Autodesk Inventor part; units mm, degrees
ref_plane "YZ Plane" through (0, 0, 0) normal (1, 0, 0) x (0, 1, 0)
ref_plane "XZ Plane" through (0, 0, 0) normal (0, 1, 0) x (-1, 0, 0)
ref_plane "XY Plane" through (0, 0, 0) normal (0, 0, 1) x (1, 0, 0)
sketch "2020_Base" plane through (0, 0, 0) normal (0, 1, 0) x (-1, 0, 0)
  line L0 (2307.7639, 1192.1343) -> (2307.7639, 1195.3915)
  arc A0 (2307.7639, 1195.3915) -> (2307.4639, 1195.6915) centre (2307.4639, 1195.3915) ccw
  line L1 (2307.4639, 1195.6915) -> (2306.5639, 1195.6915)
  arc A1 (2306.2639, 1195.9915) -> (2306.5639, 1195.6915) centre (2306.5639, 1195.9915) ccw
  line L2 (2306.2639, 1195.9915) -> (2306.2639, 1196.8915)
  arc A2 (2306.5639, 1197.1915) -> (2306.2639, 1196.8915) centre (2306.5639, 1196.8915) ccw
  line L3 (2306.5639, 1197.1915) -> (2313.3139, 1197.1915)
  arc A3 (2313.6139, 1196.8915) -> (2313.3139, 1197.1915) centre (2313.3139, 1196.8915) ccw
  line L4 (2313.6139, 1196.8915) -> (2313.6139, 1190.1415)
  arc A4 (2313.3139, 1189.8415) -> (2313.6139, 1190.1415) centre (2313.3139, 1190.1415) ccw
  line L5 (2313.3139, 1189.8415) -> (2312.4139, 1189.8415)
  arc A5 (2312.1139, 1190.1415) -> (2312.4139, 1189.8415) centre (2312.4139, 1190.1415) ccw
  line L6 (2312.1139, 1190.1415) -> (2312.1139, 1191.0415)
  arc A6 (2312.1139, 1191.0415) -> (2311.8139, 1191.3415) centre (2311.8139, 1191.0415) ccw
  line L7 (2311.8139, 1191.3415) -> (2308.5567, 1191.3415)
  arc A7 (2308.5567, 1191.3415) -> (2308.3217, 1191.2281) centre (2308.5567, 1191.0415) ccw
  arc A8 (2308.3217, 1191.2281) -> (2306.9212, 1187.4988) centre (2313.4048, 1187.1915) ccw
  line L8 (2306.9212, 1187.4988) -> (2306.6139, 1187.1915)
  line L9 (2306.6139, 1187.1915) -> (2306.9212, 1186.8843)
  arc A9 (2306.9212, 1186.8843) -> (2308.3217, 1183.155) centre (2313.4048, 1187.1915) ccw
  arc A10 (2308.3217, 1183.155) -> (2308.5567, 1183.0415) centre (2308.5567, 1183.3415) ccw
  line L10 (2308.5567, 1183.0415) -> (2311.8139, 1183.0415)
  arc A11 (2311.8139, 1183.0415) -> (2312.1139, 1183.3415) centre (2311.8139, 1183.3415) ccw
  line L11 (2312.1139, 1183.3415) -> (2312.1139, 1184.2415)
  arc A12 (2312.4139, 1184.5415) -> (2312.1139, 1184.2415) centre (2312.4139, 1184.2415) ccw
  line L12 (2312.4139, 1184.5415) -> (2313.3139, 1184.5415)
  arc A13 (2313.6139, 1184.2415) -> (2313.3139, 1184.5415) centre (2313.3139, 1184.2415) ccw
  line L13 (2313.6139, 1184.2415) -> (2313.6139, 1177.4915)
  arc A14 (2313.3139, 1177.1915) -> (2313.6139, 1177.4915) centre (2313.3139, 1177.4915) ccw
  line L14 (2313.3139, 1177.1915) -> (2306.5639, 1177.1915)
  arc A15 (2306.2639, 1177.4915) -> (2306.5639, 1177.1915) centre (2306.5639, 1177.4915) ccw
  line L15 (2306.2639, 1177.4915) -> (2306.2639, 1178.3915)
  arc A16 (2306.5639, 1178.6915) -> (2306.2639, 1178.3915) centre (2306.5639, 1178.3915) ccw
  line L16 (2306.5639, 1178.6915) -> (2307.4639, 1178.6915)
  arc A17 (2307.4639, 1178.6915) -> (2307.7639, 1178.9915) centre (2307.4639, 1178.9915) ccw
  line L17 (2307.7639, 1178.9915) -> (2307.7639, 1182.2488)
  arc A18 (2307.7639, 1182.2488) -> (2307.6505, 1182.4837) centre (2307.4639, 1182.2488) ccw
  arc A19 (2307.6505, 1182.4837) -> (2303.9212, 1183.8843) centre (2303.6139, 1177.4007) ccw
  line L18 (2303.9212, 1183.8843) -> (2303.6139, 1184.1915)
  line L19 (2303.6139, 1184.1915) -> (2303.3066, 1183.8843)
  arc A20 (2303.3066, 1183.8843) -> (2299.5774, 1182.4837) centre (2303.6139, 1177.4007) ccw
  arc A21 (2299.5774, 1182.4837) -> (2299.4639, 1182.2488) centre (2299.7639, 1182.2488) ccw
  line L20 (2299.4639, 1182.2488) -> (2299.4639, 1178.9915)
  arc A22 (2299.4639, 1178.9915) -> (2299.7639, 1178.6915) centre (2299.7639, 1178.9915) ccw
  line L21 (2299.7639, 1178.6915) -> (2300.6639, 1178.6915)
  arc A23 (2300.9639, 1178.3915) -> (2300.6639, 1178.6915) centre (2300.6639, 1178.3915) ccw
  line L22 (2300.9639, 1178.3915) -> (2300.9639, 1177.4915)
  arc A24 (2300.6639, 1177.1915) -> (2300.9639, 1177.4915) centre (2300.6639, 1177.4915) ccw
  line L23 (2300.6639, 1177.1915) -> (2293.9139, 1177.1915)
  arc A25 (2293.6139, 1177.4915) -> (2293.9139, 1177.1915) centre (2293.9139, 1177.4915) ccw
  line L24 (2293.6139, 1177.4915) -> (2293.6139, 1184.2415)
  arc A26 (2293.9139, 1184.5415) -> (2293.6139, 1184.2415) centre (2293.9139, 1184.2415) ccw
  line L25 (2293.9139, 1184.5415) -> (2294.8139, 1184.5415)
  arc A27 (2295.1139, 1184.2415) -> (2294.8139, 1184.5415) centre (2294.8139, 1184.2415) ccw
  line L26 (2295.1139, 1184.2415) -> (2295.1139, 1183.3415)
  arc A28 (2295.1139, 1183.3415) -> (2295.4139, 1183.0415) centre (2295.4139, 1183.3415) ccw
  line L27 (2295.4139, 1183.0415) -> (2298.6712, 1183.0415)
  arc A29 (2298.6712, 1183.0415) -> (2298.9061, 1183.155) centre (2298.6712, 1183.3415) ccw
  arc A30 (2298.9061, 1183.155) -> (2300.3066, 1186.8843) centre (2293.8231, 1187.1915) ccw
  line L28 (2300.3066, 1186.8843) -> (2300.6139, 1187.1915)
  line L29 (2300.6139, 1187.1915) -> (2300.3066, 1187.4988)
  arc A31 (2300.3066, 1187.4988) -> (2298.9061, 1191.2281) centre (2293.8231, 1187.1915) ccw
  arc A32 (2298.9061, 1191.2281) -> (2298.6712, 1191.3415) centre (2298.6712, 1191.0415) ccw
  line L30 (2298.6712, 1191.3415) -> (2295.4139, 1191.3415)
  arc A33 (2295.4139, 1191.3415) -> (2295.1139, 1191.0415) centre (2295.4139, 1191.0415) ccw
  line L31 (2295.1139, 1191.0415) -> (2295.1139, 1190.1415)
  arc A34 (2294.8139, 1189.8415) -> (2295.1139, 1190.1415) centre (2294.8139, 1190.1415) ccw
  line L32 (2294.8139, 1189.8415) -> (2293.9139, 1189.8415)
  arc A35 (2293.6139, 1190.1415) -> (2293.9139, 1189.8415) centre (2293.9139, 1190.1415) ccw
  line L33 (2293.6139, 1190.1415) -> (2293.6139, 1196.8915)
  arc A36 (2293.9139, 1197.1915) -> (2293.6139, 1196.8915) centre (2293.9139, 1196.8915) ccw
  line L34 (2293.9139, 1197.1915) -> (2300.6639, 1197.1915)
  arc A37 (2300.9639, 1196.8915) -> (2300.6639, 1197.1915) centre (2300.6639, 1196.8915) ccw
  line L35 (2300.9639, 1196.8915) -> (2300.9639, 1195.9915)
  arc A38 (2300.6639, 1195.6915) -> (2300.9639, 1195.9915) centre (2300.6639, 1195.9915) ccw
  line L36 (2300.6639, 1195.6915) -> (2299.7639, 1195.6915)
  arc A39 (2299.7639, 1195.6915) -> (2299.4639, 1195.3915) centre (2299.7639, 1195.3915) ccw
  line L37 (2299.4639, 1195.3915) -> (2299.4639, 1192.1343)
  arc A40 (2299.4639, 1192.1343) -> (2299.5774, 1191.8994) centre (2299.7639, 1192.1343) ccw
  arc A41 (2299.5774, 1191.8994) -> (2303.3066, 1190.4988) centre (2303.6139, 1196.9824) ccw
  line L38 (2303.3066, 1190.4988) -> (2303.6139, 1190.1915)
  line L39 (2303.6139, 1190.1915) -> (2303.9212, 1190.4988)
  arc A42 (2303.9212, 1190.4988) -> (2307.6505, 1191.8994) centre (2303.6139, 1196.9824) ccw
  arc A43 (2307.6505, 1191.8994) -> (2307.7639, 1192.1343) centre (2307.4639, 1192.1343) ccw
  circle A44 centre (2310.6139, 1194.1915) radius 2
  circle A45 centre (2303.6139, 1187.1915) radius 2.15
  circle A46 centre (2296.6139, 1194.1915) radius 2
  circle A47 centre (2296.6139, 1180.1915) radius 2
  circle A48 centre (2310.6139, 1180.1915) radius 2
  point P0 (0, 0)
extrude "500mm 2020" add sketch "2020_Base" along normal blind 500
properties part number "100mm 2020" material "알루미늄 6061"
The model under review builds one solid part; all positions refer to its coordinate system, in mm. Round coordinates to 2 decimals unless told otherwise and drop trailing zeros.
(1) We need section A-A on y = 417. Give the number of separate pieces and of enclosed holes in the cut face, and give its area (3 significant figures).
(2) Insertion check: pin 1 (3.5 mm diameter, centred on x = -2296.61, z = 1194.19, fed in from -Y). The pin has a flat end and moves straight along its axis. Give the tip position at first contact, or say it passes through.
(3) Wall thickness on L1, parallel to X at y = 338, z = 1180; L2, parallel to Z at x = -2310.25, y = 104; L3, parallel to Z at x = -2296, y = 126: over which ranges is each line inside the solid? List them lowest first.
Findings below:
1. separate pieces: 1
1. enclosed holes: 5
1. area: 146 mm2
2. pin 1: passes through
3. L1: x = -2313.61 to -2312.6, -2308.62 to -2307.76, -2299.46 to -2298.6, -2294.62 to -2293.61
3. L2: z = 1177.19 to 1178.22, 1182.16 to 1183.04, 1191.34 to 1192.22, 1196.16 to 1197.19
3. L3: z = 1177.19 to 1178.29, 1182.09 to 1183.04, 1191.34 to 1192.29, 1196.09 to 1197.19
